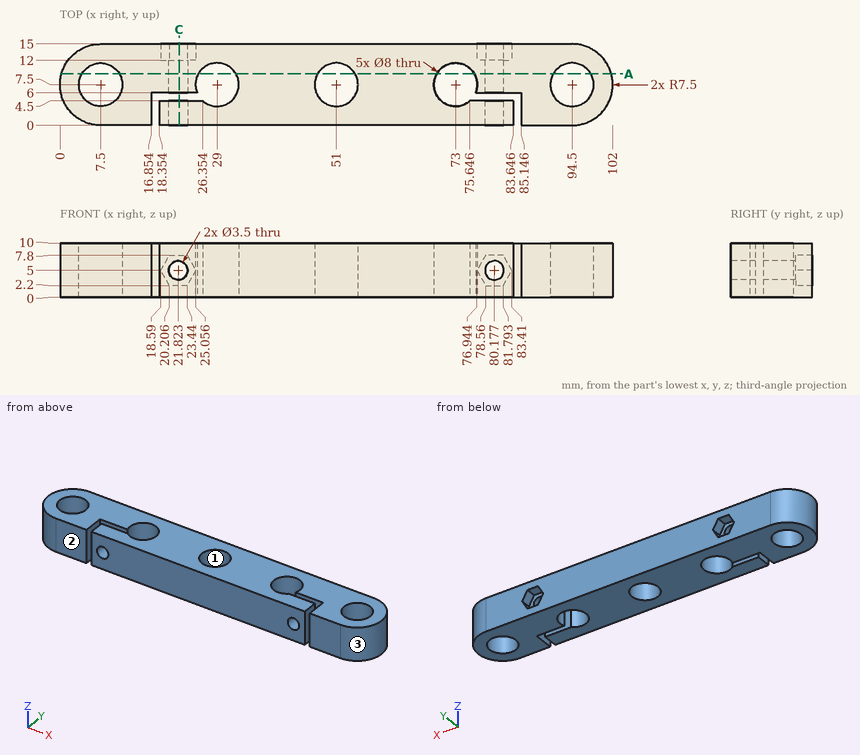
The drawing under review shows one solid part. Ordinate dimensions are in mm from its lowest x, y, z. Give positions to 0.01 mm unless a question says otherwise; leave off trailing zeros. Write each loop counter-clockwise with the first axis right and the second up, starting at its lowest first coordinate (ties: lowest second). Pieces come first, ordered by that corner, then holes. Notation, with made-up numbers: (71, -29) -> (126, -29) arc R20 cw to (126, 1) -> close; hole circle Ø2 at (-33, 27.25). An arc over 180 degrees is marked (long way). Answer in a Markdown table with one row per item.
(1) To check wall thickness, follow probe 1 along Y at (x, z) = (7.5, 3); probe 2 along X at (y, z) = (5.75, 2.75) (1 decimal); probe 3 along X at (y, z) = (12.75, 2.75) (1 decimal). State the ranges of each line that lie inside material, in increasing order.
Results:
| item | result |
|---|---|
| probe 1 | 0 to 3.5, 11.5 to 15 |
| probe 2 | 0.2 to 3.9, 11.1 to 16.9, 32.6 to 47.4, 54.6 to 69.4, 85.1 to 90.9, 98.1 to 101.8 |
| probe 3 | 2.1 to 19.9, 23.8 to 78.2, 82.1 to 99.9 |
(2) Consider section C-C (x = 22). State the section outline as (y, z) points.
Results:
| item | result |
|---|---|
| outline | (0, 0) -> (4.5, 0) -> (4.5, 3.26) -> (0, 3.26) -> close; (0, 6.74) -> (4.5, 6.74) -> (4.5, 10) -> (0, 10) -> close; (6, 0) -> (15, 0) -> (15, 2.2) -> (12, 2.2) -> (12, 3.26) -> (6, 3.26) -> close; (6, 6.74) -> (12, 6.74) -> (12, 7.8) -> (15, 7.8) -> (15, 10) -> (6, 10) -> close |
(3) Consider section A-A (y = 9.5). Count the separate pieces of the cut face and the enclosed holes in it, then the cut area to 3 significant figures.
Results:
| item | result |
|---|---|
| separate pieces | 6 |
| enclosed holes | 2 |
| area | 649 mm2 |
(4) Clearance check with flat-ended pins moving along their axes: pin 1 (1 mm diameter, centred on y = 8.5, z = 8.5, fed in from -X); pin 2 (3 mm diameter, centred on y = 2, z = 4.5, fed in from -X) (1 decimal); pin 3 (2 mm diameter, centred on y = 2.5, z = 3.5, fed in from +X) (1 decimal). State where each tip first meets the part, or that it passes through.
Results:
| item | result |
|---|---|
| pin 1 | x = 0.02 |
| pin 2 | x = 1.2 |
| pin 3 | x = 100.8 |
(5) Mouldability with a two-part tool opening along X and no side actions: class the marked faces 1, 2 and 3 as +X half, -X half, draft (parallel to the pull), parting line (faces both ways), or undercut.
Results:
| item | result |
|---|---|
| face 1 | undercut |
| face 2 | draft |
| face 3 | +X half |
